Check sheet for the drawn part. Datum: minimum x, y, z corner. Units: mm. A direction names the side the tool comes from. Round coordinates to 2 decimals unless told otherwise and drop trailing zeros. Order: outer loops, then holes, each group sorted by start corner. A loop starts at its lowest first (then second) coordinate and runs counter-clockwise, first axis right, second up. Notation, with made-up numbers: (-12.5, 7) - (33.5, 7) arc R18 cw to (33.5, 34) - close; hole circle Ø7 at (-10, 64). An arc over 180 degrees is marked (long way). Write each question's results on one line, items separated by ' | '.
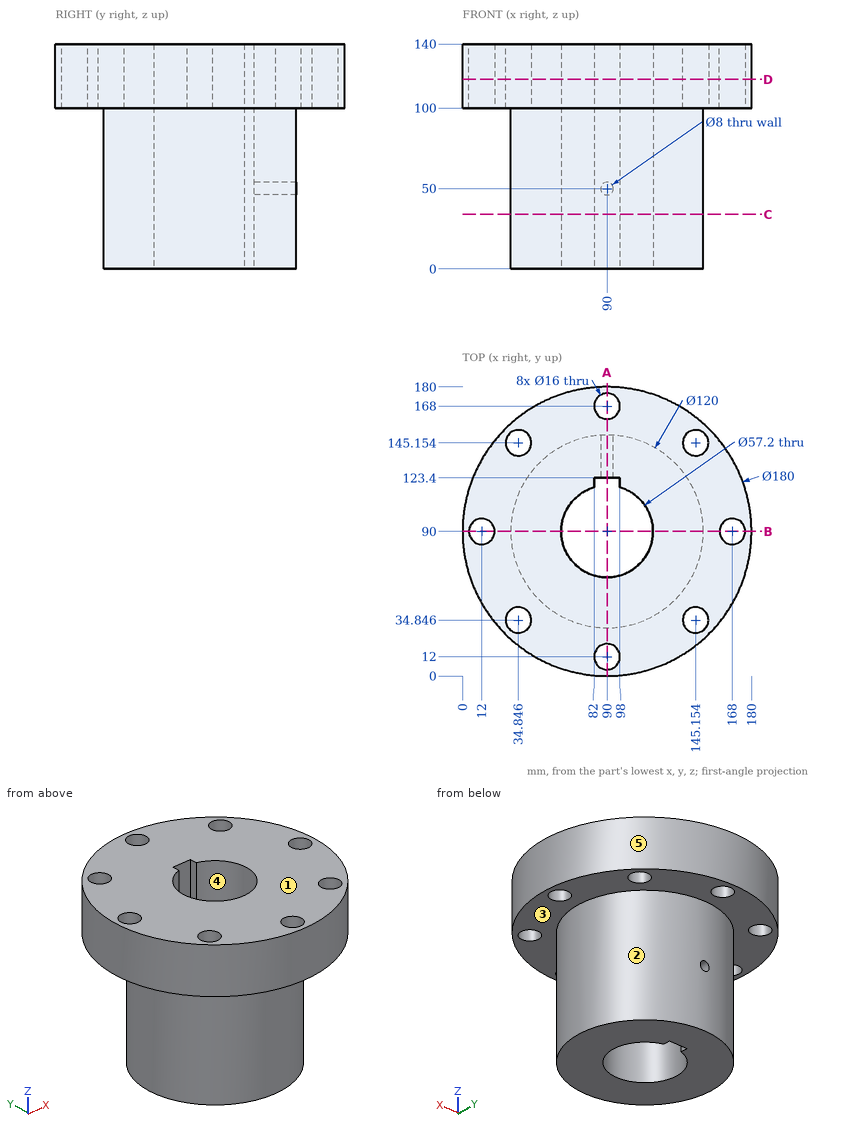
(1) Section check B-B (y = 90). Record the cut outline in (x, z).
Answers follow:
outline: (0, 100) - (4, 100) - (4, 140) - (0, 140) - close; (20, 100) - (30, 100) - (30, 0) - (61.4, 0) - (61.4, 140) - (20, 140) - close; (118.6, 0) - (150, 0) - (150, 100) - (160, 100) - (160, 140) - (118.6, 140) - close; (176, 100) - (180, 100) - (180, 140) - (176, 140) - close
(2) Section check A-A (x = 90). Record the cut outline in (y, z).
Answers follow:
outline: (0, 100) - (4, 100) - (4, 140) - (0, 140) - close; (20, 100) - (30, 100) - (30, 0) - (61.4, 0) - (61.4, 140) - (20, 140) - close; (123.4, 0) - (150, 0) - (150, 46) - (123.4, 46) - close; (123.4, 54) - (150, 54) - (150, 100) - (160, 100) - (160, 140) - (123.4, 140) - close; (176, 100) - (180, 100) - (180, 140) - (176, 140) - close
(3) Access from +Z, -Z, +X, -X, +Y, -Y to the whole of each face (thin tool, end or side, straight path). Record for the marked faces 1 and 2.
Answers follow:
face 1: +Z, +X, -X, +Y, -Y | face 2: -Z
(4) Material ranges on line 1 (Y direction, x = 86.5, z = 108) (1 decimal); line 2 (Z direction, x = 90, y = 142); line 3 (Y direction, x = 110, z = 52) (1 decimal), recorded low to high.
Answers follow:
line 1: 0.1 to 4.8, 19.2 to 61.6, 123.4 to 160.8, 175.2 to 179.9 | line 2: 0 to 46, 54 to 140 | line 3: 33.4 to 69.6, 110.4 to 146.6
(5) Section check C-C (z = 34). Record the cut outline in (x, y).
Answers follow:
outline: circle Ø120 at (90, 90); hole (82, 117.46) arc R28.6 ccw (long way) to (98, 117.46) - (98, 123.4) - (82, 123.4) - close
(6) Draft check along X on the marked faces 3, 4 and 5. Enter one of: released by +X, released by -X, zero draft, split by the parting line, or undercut.
Answers follow:
face 3: zero draft | face 4: undercut | face 5: split by the parting line
(7) Section check D-D (z = 118). Give the number of separate pieces and of enclosed holes in the cut face, then the cut area to 3 significant figures.
Answers follow:
separate pieces: 1 | enclosed holes: 9 | area: 21,200 mm²
(8) Depth check by flat-ended pin: pin 1 Ø3 at (x, y) = (55.5, 24.5) entering from -Z; pin 2 Ø18.5 at (x, y) = (12, 90) entering from +Z; pin 3 Ø3 at (y, z) = (119, 101.5) entering from -X; pin 4 Ø13 at (x, z) = (90, 50) entering from +Y. Enter the tip coordinate at first touch or a pass-through.
Answers follow:
pin 1: z = 100 | pin 2: z = 140 | pin 3: x = 4.3 | pin 4: y = 150
